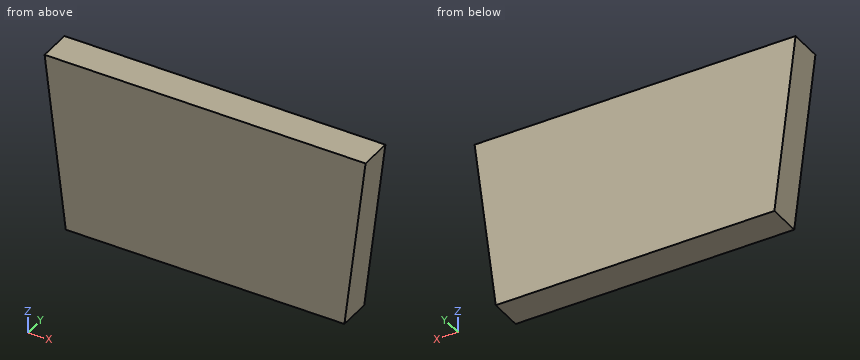
from build123d import *

# Parameters (mm, degrees)
SALIENTE_EXTRUIR1_DEPTH = 30
CORTAR_EXTRUIR2_DEPTH   = 90
CROQUIS5_W              = 20
CROQUIS5_H              = 2
SALIENTE_EXTRUIR2_DEPTH = 3
CHAFL_N1_SIZE           = 15
CHAFL_N1_SIZE2          = 4.585960222
CHAFL_N2_SIZE           = 15
CHAFL_N2_SIZE2          = 4.585960222
CHAFL_N3_SIZE           = 15
CHAFL_N3_SIZE2          = 4.873795443
SALIENTE_EXTRUIR3_DEPTH = 5
CROQUIS7_W              = 20
CROQUIS7_H              = 2
CORTAR_EXTRUIR3_DEPTH   = 65
CROQUIS8_W              = 69.078643268
CROQUIS8_H              = 63.245130673
CORTAR_EXTRUIR4_DEPTH   = 5


with BuildPart() as part:
    # Croquis2 → Saliente-Extruir1 (new body)
    with BuildSketch(Plane(origin=(0, 0, 0), x_dir=(1, 0, 0), z_dir=(0, 1, 0))):
        Polygon((0, 0), (4.293050572, 35.408576274), (-0.206949428, 35.33296049), (-14, 0), align=None)
        Polygon((24.793050572, 35.408576274), (4.293050572, 35.408576274), (3.44434788, 28.408576274), (24.793050572, 28.408576274), align=None)
        Polygon((45.293050572, 35.408576274), (24.793050572, 35.408576274), (24.793050572, 28.408576274), (46.141753264, 28.408576274), align=None)
        Polygon((49.793050572, 35.33296049), (63.586101144, 0), (49.586101144, 0), (45.293050572, 35.408576274), align=None)
    extrude(amount=SALIENTE_EXTRUIR1_DEPTH)

    # Croquis4 → Cortar-Extruir2 (cut, symmetric)
    with BuildSketch(Plane(origin=(0, 0, 0), x_dir=(0, 0, -1), z_dir=(1, 0, 0))):
        Polygon((0, 0), (5, 0), (5, 30), (-4.90661078, 30), (-4.90661078, 0), align=None)
    extrude(amount=CORTAR_EXTRUIR2_DEPTH, both=True, mode=Mode.SUBTRACT)

    # Croquis5 → Saliente-Extruir2 (add)
    with BuildSketch(Plane(origin=(0, 0, 0), x_dir=(-1, 0, 0), z_dir=(0, -1, 0))):
        with Locations((-24.793050572, 32.408576274)):
            Rectangle(CROQUIS5_W, CROQUIS5_H)
    extrude(amount=SALIENTE_EXTRUIR2_DEPTH)

    # Chaflán1
    chafl_n1_edges = [part.edges().sort_by_distance(p)[0] for p in [
        (2.025282044, 30, -16.704288137),
    ]]
    chafl_n1_side = [part.faces().sort_by_distance(p)[0] for p in [
        (2.025282044, 15, -16.704288137),
    ]]
    chamfer(chafl_n1_edges, length=CHAFL_N1_SIZE, length2=CHAFL_N1_SIZE2, reference=chafl_n1_side[0])

    # Chaflán2
    chafl_n2_edges = [part.edges().sort_by_distance(p)[0] for p in [
        (47.5608191, 30, -16.704288137),
    ]]
    chafl_n2_side = [part.faces().sort_by_distance(p)[0] for p in [
        (47.5608191, 15, -16.704288137),
    ]]
    chamfer(chafl_n2_edges, length=CHAFL_N2_SIZE, length2=CHAFL_N2_SIZE2, reference=chafl_n2_side[0])

    # Chaflán3
    chafl_n3_edges = [part.edges().sort_by_distance(p)[0] for p in [
        (24.793050572, 30, -28.408576274),
    ]]
    chafl_n3_side = [part.faces().sort_by_distance(p)[0] for p in [
        (24.793050572, 15.5132008, -28.408576274),
    ]]
    chamfer(chafl_n3_edges, length=CHAFL_N3_SIZE, length2=CHAFL_N3_SIZE2, reference=chafl_n3_side[0])

    # Croquis7 → Cortar-Extruir3 (cut)
    # profile 1 of 3: a face of its own
    with BuildSketch(Plane.XZ):
        Polygon((0.606216209, -38.306494664), (49.793050572, -38.306494664), (49.793050572, -35.33296049), (45.293050572, -35.408576274), (4.293050572, -35.408576274), (-0.206949428, -35.33296049), align=None)
    # profile 2 of 3: a face of its own
    with BuildSketch(Plane.XZ):
        Polygon((-0.206949428, -35.33296049), (49.793050572, -35.33296049), (61.634233768, -5), (48.979884935, -5), (46.141753264, -28.408576274), (3.44434788, -28.408576274), (0.606216209, -5), (-12.048132625, -5), align=None)
        with Locations((24.793050572, -32.408576274)):
            Rectangle(CROQUIS7_W, CROQUIS7_H, mode=Mode.SUBTRACT)
    # profile 3 of 3: a face of its own
    with BuildSketch(Plane.XZ):
        with Locations((24.793050572, -32.408576274)):
            Rectangle(CROQUIS7_W, CROQUIS7_H)
    extrude(amount=-CORTAR_EXTRUIR3_DEPTH, mode=Mode.SUBTRACT)


with BuildPart() as body_2:
    # Croquis6 → Saliente-Extruir3 (new body)
    with BuildSketch(Plane.XZ):
        Polygon((0.608725752, -1.697385274), (3.798779842, -28.008576274), (45.787321302, -28.008576274), (48.977375392, -1.697385274), align=None)
    extrude(amount=-SALIENTE_EXTRUIR3_DEPTH)


with BuildPart() as cortar_extruir3_piece_1:
    # of the separate pieces the step leaves, piece 1, a body of its own (cortar_extruir3_pieces)
    add(part.part.solids().sort_by_distance((14.793050572, 0, -31.408576274))[0])


with BuildPart() as cortar_extruir3_piece_2:
    # of the separate pieces the step leaves, piece 2, a body of its own (cortar_extruir3_pieces)
    add(part.part.solids().sort_by_distance((4.293050572, 0, -35.408576274))[0])


with BuildPart() as cortar_extruir4_tool:
    # Croquis8 → Cortar-Extruir4 (new body)
    with BuildSketch(Plane(origin=(0, 0, -35.408576274), x_dir=(-1, 0, 0), z_dir=(0, 0, -1))):
        with Locations((-28.687723689, 10.469966138)):
            Rectangle(CROQUIS8_W, CROQUIS8_H)
    extrude(amount=-CORTAR_EXTRUIR4_DEPTH)


with BuildPart() as cortar_extruir3_piece_1_1:
    add(cortar_extruir3_piece_1.part)

    # Cortar-Extruir4: cut by cortar_extruir4_tool
    add(cortar_extruir4_tool.part, mode=Mode.SUBTRACT)


with BuildPart() as cortar_extruir3_piece_2_1:
    add(cortar_extruir3_piece_2.part)

    # Cortar-Extruir4: cut by cortar_extruir4_tool
    add(cortar_extruir4_tool.part, mode=Mode.SUBTRACT)


solid = body_2.part
Here's how the part is built. I have some questions about the finished solid (model axes, mm). Coordinates: 2 decimals unless noted, no trailing zeros. Order: outer loops, then holes, each group sorted by start corner. A loop starts at its lowest first (then second) coordinate and runs counter-clockwise, first axis right, second up. Notation, with made-up numbers: (-29.75, 14) - (3.25, 14) arc R28 cw to (3.25, 32) - close; hole circle Ø10 at (55, -35.5). An arc over 180 degrees is marked (long way). Use CSV: the item, a comma, the result in double quotes. Start each with the question number.
1. Suppose I cut it at B-B on z = -16.5. List the corners of the cut face in (x, y) for me, then the cut area to 3 significant figures.
2. Please list where these lines run through material, in increasing order: line 1 (X direction, y = 2, z = -24); line 2 (X direction, y = 0.35, z = -5.5). Write a range as from..to.
3. Suppose I cut it at A-A on y = 1.1. List the corners of the cut face in (x, z) for me.
4. I'm going to push flat-ended pins straight in: pin 1 (1.5 mm diameter, centred on y = 3.5, z = -19.5, fed in from -X); pin 2 (10 mm diameter, centred on x = 43.5, z = -6.5, fed in from -Y). Where does each tip first touch, or does it pass through?
Output:
1,outline,"(2.4, 0) - (47.18, 0) - (47.18, 5) - (2.4, 5) - close"
1,area,"224 mm2"
2,line 1,"x = 3.31..46.27"
2,line 2,"x = 1.07..48.52"
3,outline,"(0.61, -1.7) - (3.8, -28.01) - (45.79, -28.01) - (48.98, -1.7) - close"
4,pin 1,"stops at x = 2.68"
4,pin 2,"stops at y = 0"
